from build123d import *

# Parameters (mm, degrees)
F0_W     = 318
F0_H     = 130
F1_DEPTH = 5
F2_R     = 20
F3_T     = -2


with BuildPart() as f1:
    # F0 (on Front) → F1 (new body)
    with BuildSketch(Plane.XZ):
        Rectangle(F0_W, F0_H)
    extrude(amount=F1_DEPTH)

    # F2
    f2_edges = [f1.edges().sort_by_distance(p)[0] for p in [
        (-159, -2.5, -65),
        (159, -2.5, -65),
        (159, -2.5, 65),
        (-159, -2.5, 65),
    ]]
    fillet(f2_edges, radius=F2_R)

    # F3
    f3_openings = [f1.faces().sort_by_distance(p)[0] for p in [
        (0, -5, 0),
        (0, 0, 0),
    ]]
    offset(amount=F3_T, openings=f3_openings)


solid = f1.part
Check sheet for the modelled part. Datum: model origin and axes. Units: mm. A direction names the side the tool comes from. Round coordinates to 2 decimals unless told otherwise and drop trailing zeros. Order: outer loops, then holes, each group sorted by start corner. A loop starts at its lowest first (then second) coordinate and runs counter-clockwise, first axis right, second up.
Q1. Draft check along Z on faces 1 (the face through (152.986, -2.535, -59.297)), 2 (the face through (151.867, -2.535, 57.587)), 3 (the face through (-151.867, -2.535, -57.587)), 4 (the face through (153.297, -2.535, 58.986)). Enter one of: pulls with the +Z half, pulls with the -Z half, needs draft (parallel to the pull), parting line crosses it, or undercut.
Filled sheet:
face 1: pulls with the -Z half
face 2: undercut
face 3: undercut
face 4: pulls with the +Z half
Q2. Scan lines: L1, parallel to Z at x = 139, y = -2.45; L2, parallel to X at y = -3.75, z = -18; L3, parallel to X at y = -2.7, z = -57.5. Record each from-to range of solid material in increasing order.
Filled sheet:
L1: z = -65 to -63, 63 to 65
L2: x = -159 to -157, 157 to 159
L3: x = -154.61 to -151.95, 151.95 to 154.61
Q3. Cross-section at C-C, the plane y = -4.1. Enter the section's corners in (x, z), plus the area to 3 significant figures.
Filled sheet:
outline: (-159, -45) arc R20 ccw to (-139, -65) - (139, -65) arc R20 ccw to (159, -45) - (159, 45) arc R20 ccw to (139, 65) - (-139, 65) arc R20 ccw to (-159, 45) - close; hole (-157, -45) arc R18 ccw to (-139, -63) - (139, -63) arc R18 ccw to (157, -45) - (157, 45) arc R18 ccw to (139, 63) - (-139, 63) arc R18 ccw to (-157, 45) - close
area: 1,710 mm2
Q4. Cross-section at B-B, the plane x = 46.5. Enter the section's corners in (y, z), plus the area to 3 significant figures.
Filled sheet:
outline: (-5, -65) - (0, -65) - (0, -63) - (-5, -63) - close; (-5, 63) - (0, 63) - (0, 65) - (-5, 65) - close
area: 20.0 mm2
Q5. Cross-section at A-A, the plane z = 4.5. Enter the section's corners in (x, y).
Filled sheet:
outline: (-159, -5) - (-157, -5) - (-157, 0) - (-159, 0) - close; (157, -5) - (159, -5) - (159, 0) - (157, 0) - close
Q6. Set-up check for faces 5 (the face through (151.587, -2.535, -57.867)), 6 (the face through (-153.297, -2.535, 58.986)): record each of +Z, -Z, +X, -X, +Y, -Y from which the full face is reachable in a straight line by a thin tool's end or side.
Filled sheet:
face 5: +Y, -Y
face 6: +Z, -X, +Y, -Y
